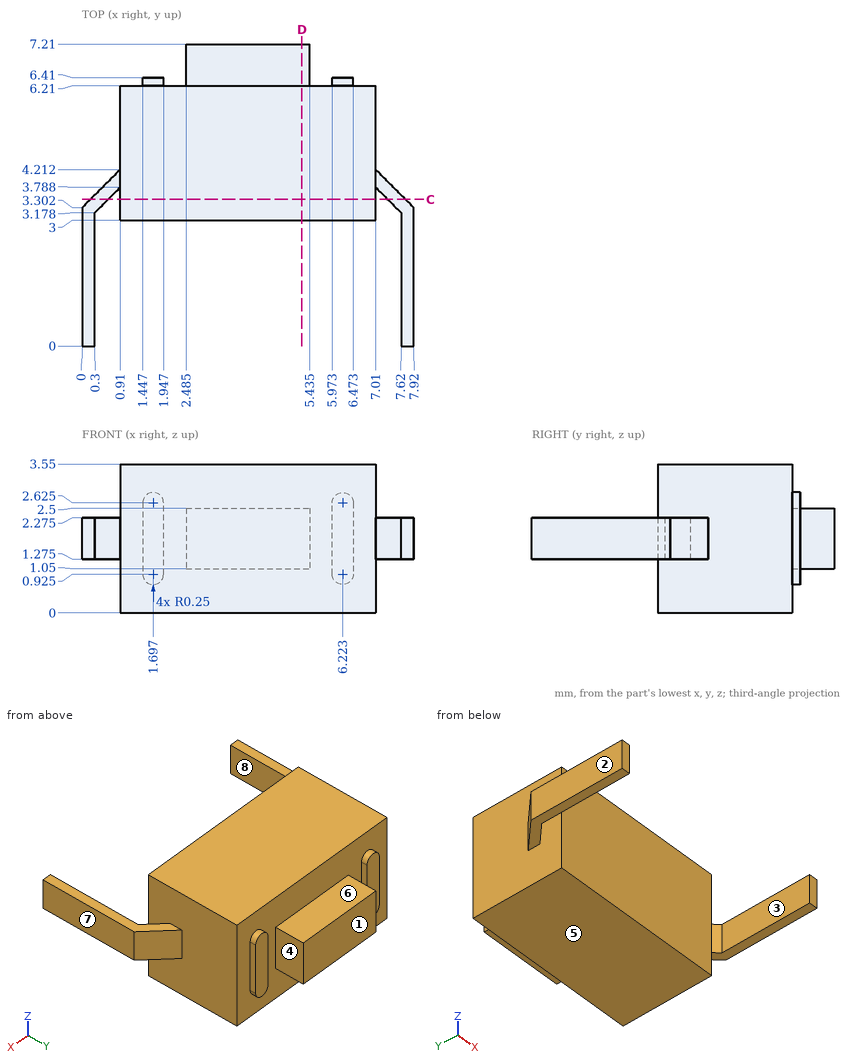
Answer from the drawing. Dimensions are ordinates in mm from the lowest x, y and z of the part. A direction names the side the tool comes from. Give positions to 0.01 mm unless a question says otherwise; leave off trailing zeros. Loops run counter-clockwise (first coordinate to the right, second up) from the corner with the lowest first, then second, coordinate; pieces in that order, holes last.
Item 1: Find the intervals of material crossed by line 1 along Z through (x, y) = (5, 6.25); line 2 along X through (y, z) = (1.5, 2.15); line 3 along Y through (x, z) = (4.75, 1.55), in increasing order.
Item 2: For the marked faces 4, 5, 6, 7 and 8, determine the directions among +Z, -Z, +X, -X, +Y, -Y from which every point of the face is accessible in a straight line to the end or side of a thin tool.
Item 3: Each of these flat-tipped pins is pushed along its axis until it touches: pin 1 Ø1.1 at (x, z) = (4, 2) entering from -Y; pin 2 Ø4 at (x, y) = (3, 2) entering from -Z; pin 3 Ø3 at (x, y) = (3.5, 1) entering from +Z; pin 4 Ø1.6 at (y, z) = (4.5, 2.5) entering from +X. Where does it stop, or does it pass through?
Item 4: The part is cut by section C-C (y = 3.5). Give the number of separate pieces and of enclosed holes in the cut face, and give its area (3 significant figures).
Item 5: The part is cut by section D-D (x = 5.25). Write down the section's boundary in (y, z).
Item 6: The mould has two halves that part along X. Classify the marked faces 1, 2 and 3: released by +X, released by -X, zero draft, split by the parting line, or undercut.
Taken from the geometry:
1. line 1: z = 1.05 to 2.5
1. line 2: x = 0 to 0.3, 7.62 to 7.92
1. line 3: y = 3 to 7.21
2. face 4: +Z, -Z, +Y
2. face 5: -Z, +X, -X, +Y, -Y
2. face 6: +Z, +Y
2. face 7: +Z, -Z, +X, +Y, -Y
2. face 8: +Z, -Z, -Y
3. pin 1: stops at y = 3
3. pin 2: stops at z = 0
3. pin 3: passes through
3. pin 4: stops at x = 7.49
4. separate pieces: 3
4. enclosed holes: 0
4. area: 22.5 mm2
5. outline: (3, 0) - (6.21, 0) - (6.21, 1.05) - (7.21, 1.05) - (7.21, 2.5) - (6.21, 2.5) - (6.21, 3.55) - (3, 3.55) - close
6. face 1: zero draft
6. face 2: released by -X
6. face 3: undercut
